Could you check a few things on this model? Use its own coordinates, in mm. A direction names the side the tool comes from. Round coordinates to 2 decimals unless told otherwise and drop trailing zeros. Order: outer loops, then holes, each group sorted by start corner. A loop starts at its lowest first (then second) coordinate and runs counter-clockwise, first axis right, second up. Notation, with made-up numbers: (12, -7) -> (17, -7) arc R28 ccw to (17, 27) -> close; hole circle Ø1 at (85, -11.5). An arc over 180 degrees is marked (long way). Put each result on its own line as item: value. Start each with the question number.
from build123d import *

# Parameters (mm, degrees)
SKETCH_1_W          = 22.5
SKETCH_1_H          = 20
EXTRUDE_1_DEPTH     = 20
SKETCH_2_W          = 20
SKETCH_2_H          = 4.25
EXTRUDE_2_DEPTH     = 5
SKETCH_3_R          = 1.5
CUT_EXTRUDE_1_DEPTH = 32.721443851
SKETCH_4_W          = 27.5
SKETCH_4_H          = 20
EXTRUDE_3_DEPTH     = 10
SKETCH_5_R          = 1.25
CUT_EXTRUDE_2_DEPTH = 15
CHAMFER_1_SIZE      = 1.5


with BuildPart() as part:
    # 草图1 → 凸台-拉伸1 (new body)
    with BuildSketch(Plane(origin=(0, 0, 0), x_dir=(1, 0, 0), z_dir=(0, 1, 0))):
        Rectangle(SKETCH_1_W, SKETCH_1_H)
    extrude(amount=EXTRUDE_1_DEPTH)

    # 草图2 → 凸台-拉伸2 (add)
    with BuildSketch(Plane(origin=(11.25, 0, 0), x_dir=(0, 0, -1), z_dir=(1, 0, 0))):
        with Locations((0, 17.875)):
            Rectangle(SKETCH_2_W, SKETCH_2_H)
        with Locations((0, 2.125)):
            Rectangle(SKETCH_2_W, SKETCH_2_H)
    extrude(amount=EXTRUDE_2_DEPTH)

    # 草图3 → 切除-拉伸1 (cut, through all)
    with BuildSketch(Plane(origin=(11.25, 0, 0), x_dir=(0, 0, -1), z_dir=(1, 0, 0))):
        with Locations((6.496047989, 10)):
            Circle(SKETCH_3_R)
        with Locations((-6.496047989, 10)):
            Circle(SKETCH_3_R)
    extrude(amount=-CUT_EXTRUDE_1_DEPTH, mode=Mode.SUBTRACT)

    # 草图4 → 凸台-拉伸3 (add)
    with BuildSketch(Plane(origin=(0, 20, 0), x_dir=(1, 0, 0), z_dir=(0, 1, 0))):
        with Locations((2.5, 0)):
            Rectangle(SKETCH_4_W, SKETCH_4_H)
    extrude(amount=EXTRUDE_3_DEPTH)

    # 草图5 → 切除-拉伸2 (cut)
    with BuildSketch(Plane(origin=(0, 30, 0), x_dir=(1, 0, 0), z_dir=(0, 1, 0))):
        with Locations(Location((6.25, 6.25, 0), (0, 0, 270))):
            Circle(SKETCH_5_R)
        with Locations(Location((6.25, -6.25, 0), (0, 0, 270))):
            Circle(SKETCH_5_R)
        with Locations(Location((-6.25, 6.25, 0), (0, 0, 270))):
            Circle(SKETCH_5_R)
        with Locations(Location((-6.25, -6.25, 0), (0, 0, 270))):
            Circle(SKETCH_5_R)
    extrude(amount=-CUT_EXTRUDE_2_DEPTH, mode=Mode.SUBTRACT)

    # 倒角1
    chamfer_1_edges = [part.edges().sort_by_distance(p)[0] for p in [
        (16.25, 22.875, 10),
        (16.25, 22.875, -10),
        (16.25, 2.125, -10),
        (16.25, 2.125, 10),
        (2.5, 0, -10),
        (2.5, 0, 10),
        (-11.25, 0, 0),
        (-11.25, 15, -10),
        (-11.25, 15, 10),
    ]]
    chamfer(chamfer_1_edges, length=CHAMFER_1_SIZE)


solid = part.part
1. For pin 1 Ø6 at (y, z) = (7.5, -2) entering from +X; pin 2 Ø2.5 at (y, z) = (10, 6.5) entering from -X; pin 3 Ø0.8 at (x, z) = (6, 6) entering from +Y, each with a flat end and sliding along its axis, tell me the tip position at first contact or that it passes through.
2. If we section it at A-A, the plane x = 7: Please give me the cut outline in (y, z), then the cut area to 3 significant figures.
3. Thinking about a two-plate mould opening in X: for faces 4 (the face through (-10.49, 15.95, -9.26)), 5 (the face through (3, 0, 0)), 6 (the face through (-7.01, 22.6, -7.24)), 7 (the face through (15.51, 22.78, 9.24)), which applies, +X half, -X half, draft (parallel to the pull), parting line (faces both ways), or undercut?
4. If we section it at B-B, the plane z = -6.25: Please give me the cut outline in (x, y), then the cut area to 3 significant figures.
5. If we section it at C-C, the plane z = -4: Please give me the cut outline in (x, y).
6. Which directions (+Z, -Z, +X, -X, +Y, -Y) give clear straight access to the entire face, cutting with the end or side of a thin tool? Please do faces 1 (the face through (-6, 15, -6)), 2 (the face through (11.25, 10, 0)), 3 (the face through (15.51, 22.97, -9.24)).
7. I need wall thicknesses on L1, parallel to X at y = 22.5, z = -6.25; L2, parallel to Y at x = 14.5, z = 5; L3, parallel to Z at x = -4.75, y = 11. Which ranges of each line are inside material? Lowest first, please.
8. If we section it at D-D, the plane y = 5: Please give me the cut outline in (x, z).
Results below:
1. pin 1: x = 11.25
1. pin 2: through
1. pin 3: y = 15
2. outline: (0, -8.5) -> (1.5, -10) -> (30, -10) -> (30, -7.25) -> (15, -7.25) -> (15, -5.25) -> (30, -5.25) -> (30, 5.25) -> (15, 5.25) -> (15, 7.25) -> (30, 7.25) -> (30, 10) -> (1.5, 10) -> (0, 8.5) -> close; hole circle Ø3 at (10, -6.5); hole circle Ø3 at (10, 6.5)
2. area: 524 mm2
3. face 4: -X half
3. face 5: draft
3. face 6: undercut
3. face 7: +X half
4. outline: (-11.25, 1.5) -> (-9.75, 0) -> (16.25, 0) -> (16.25, 4.25) -> (11.25, 4.25) -> (11.25, 8.52) -> (-11.25, 8.52) -> close; (-11.25, 11.48) -> (11.25, 11.48) -> (11.25, 15.75) -> (16.25, 15.75) -> (16.25, 30) -> (7.5, 30) -> (7.5, 15) -> (5, 15) -> (5, 30) -> (-5, 30) -> (-5, 15) -> (-7.5, 15) -> (-7.5, 30) -> (-11.25, 30) -> close
4. area: 625 mm2
5. outline: (-11.25, 1.5) -> (-9.75, 0) -> (16.25, 0) -> (16.25, 4.25) -> (11.25, 4.25) -> (11.25, 15.75) -> (16.25, 15.75) -> (16.25, 30) -> (-11.25, 30) -> close
6. face 1: +Y
6. face 2: +Z, -Z, +X
6. face 3: -Z, +X, +Y, -Y
7. L1: -11.25 to -7.5, -5 to 5, 7.5 to 16.25
7. L2: 0 to 4.25, 15.75 to 30
7. L3: -10 to -7.61, -5.38 to 5.38, 7.61 to 10
8. outline: (-11.25, -8.5) -> (-9.75, -10) -> (11.25, -10) -> (11.25, 10) -> (-9.75, 10) -> (-11.25, 8.5) -> close
